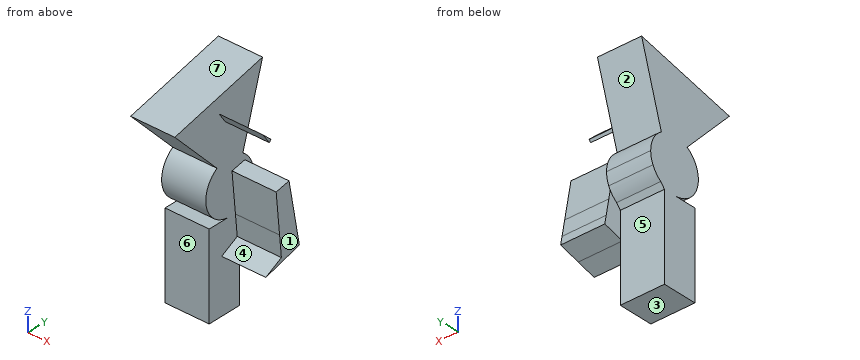
```python
from build123d import *

# Parameters (mm, degrees)
F1_DEPTH = 25.4
F3_DEPTH = 25.4


with BuildPart() as f1:
    # F0 (on Right) → F1 (new body)
    with BuildSketch(Plane.YZ):
        Polygon((-13.2883740589, -47.1408768902), (-13.2883740589, -64.2038285732), (6.5742493607, -64.2038285732), (6.5742493607, -19.7971570041), (0, -15.5264167115), (-13.2883740589, -15.5264167115), align=None)
        Polygon((0, -15.5264167115), (6.5742493607, -19.7971570041), (6.5742493607, -15.5264167115), align=None)
        with BuildLine():
            Line((0, -15.5264167115), (6.5742493607, -15.5264167115))
            Line((6.5742493607, -15.5264167115), (8.9490753187, -12.6879339074))
            ThreePointArc((8.9490753187, -12.6879339074), (4.6942234099, -14.7997933255), (0, -15.5264167115))
        make_face()
        with BuildLine():
            ThreePointArc((-8.216208845, 13.1743511459), (-14.9268228651, -4.2731224008), (0, -15.5264167115))
            ThreePointArc((0, -15.5264167115), (4.6942234099, -14.7997933255), (8.9490753187, -12.6879339074))
            Line((8.9490753187, -12.6879339074), (14.0681090783, -6.5694689939))
            ThreePointArc((14.0681090783, -6.5694689939), (15.1574559177, -3.3646910711), (15.5264167115, 0))
            ThreePointArc((15.5264167115, 0), (13.6875468883, 7.3294390017), (8.6065101962, 12.9227550523))
            Line((8.6065101962, 12.9227550523), (4.6159664635, -0.419639051))
            Line((4.6159664635, -0.419639051), (-8.216208845, 13.1743511459))
        make_face()
        with BuildLine():
            Line((14.0681090783, -6.5694689939), (8.9490753187, -12.6879339074))
            ThreePointArc((8.9490753187, -12.6879339074), (11.908257539, -9.9630827701), (14.0681090783, -6.5694689939))
        make_face()
        with BuildLine():
            Line((-35.7222311496, 42.3133387746), (-8.216208845, 13.1743511459))
            ThreePointArc((-8.216208845, 13.1743511459), (0.2321829769, 15.5246805753), (8.6065101962, 12.9227550523))
            Line((8.6065101962, 12.9227550523), (21.4547120332, 55.8807537376))
            Line((21.4547120332, 55.8807537376), (-35.7222311496, 42.3133387746))
        make_face()
        with BuildLine():
            ThreePointArc((8.6065101962, 12.9227550523), (0.2321829769, 15.5246805753), (-8.216208845, 13.1743511459))
            Line((-8.216208845, 13.1743511459), (4.6159664635, -0.419639051))
            Line((4.6159664635, -0.419639051), (8.6065101962, 12.9227550523))
        make_face()
    extrude(amount=F1_DEPTH)

    # F2 (on face) → F3 (join)
    with BuildSketch(Plane.YZ.offset(25.4)):
        Polygon((-2.8975114851, 34.5519260837), (-1.9047569793, 35.8120341569), (-6.9570055408, 40.475821833), align=None)
        Polygon((9.9313091487, 8.8122906163), (1.5386517625, 7.1337586269), (3.7782862439, -16.0091173098), (14.0347183236, -13.2288791008), align=None)
        Polygon((14.0347183236, -13.2288791008), (3.7782862439, -16.0091173098), (4.9502783877, -28.1196956248), (15.7521614301, -22.4540022549), align=None)
        Polygon((15.7521614301, -22.4540022549), (4.9502783877, -28.1196956248), (5.1841876849, -30.5367569319), (16.6601009867, -27.330934827), align=None)
        Polygon((5.1841876849, -30.5367569319), (4.9502783877, -28.1196956248), (-5.1754731685, -33.4307514131), align=None)
    extrude(amount=F3_DEPTH)


solid = f1.part
```
Verification items for the finished model (mm, model axes). Face numbers are marked on the shaded views. A direction names the side the tool comes from. Give positions to 0.01 mm unless a question says otherwise; leave off trailing zeros. Loops run counter-clockwise (first coordinate to the right, second up) from the corner with the lowest first, then second, coordinate; pieces in that order, holes last.
1. Set-up check for the marked faces 5, 6 and 7: record each of +Z, -Z, +X, -X, +Y, -Y from which the full face is reachable in a straight line by a thin tool's end or side.
2. Section check A-A, the plane x = 39.5. Enter the section's corners in (y, z), then the cut area to 3 significant figures.
3. Thickness scan on line 1 (Y direction, x = 18.5, z = -21); line 2 (X direction, y = -11, z = -5.5); line 3 (Z direction, x = 17, y = -24). Record the ranges inside material, lowest first.
4. Section check D-D, the plane y = -21. Enter the section's corners in (x, z), then the cut area to 3 significant figures.
5. Mould release check, pull along Z, two halves, no side actions. Record for the marked faces 1, 2, 3 and 4: released by +Z, released by -Z, zero draft, split by the parting line, or undercut.
6. Go/stop test with flat-tipped pins: pin 1 Ø4 at (x, y) = (14.5, -12.5) entering from +Z; pin 2 Ø1.5 at (x, z) = (12, -22.5) entering from -Y; pin 3 Ø4 at (x, y) = (17, -26) entering from -Z. Record where each tip stops, or that it passes through.
7. Section check C-C, the plane x = 23.5. Enter the section's corners in (y, z), then the cut area to 3 significant figures.
8. Section check B-B, the plane z = 38.5. Enter the section's corners in (x, y).
Geometry says:
1. face 5: -Z, -X, +Y
1. face 6: -Z, +X, -X, -Y
1. face 7: +Z, +X, -X, -Y
2. outline: (-6.96, 40.48) - (-2.9, 34.55) - (-1.9, 35.81) - close; (-5.18, -33.43) - (16.66, -27.33) - (9.93, 8.81) - (1.54, 7.13) - (4.95, -28.12) - close
2. area: 398 mm2
3. line 1: y = -13.29 to 6.57
3. line 2: x = 0 to 25.4
3. line 3: z = 29.9 to 45.09
4. outline: (0, 26.72) - (25.4, 26.72) - (25.4, 45.81) - (0, 45.81) - close
4. area: 485 mm2
5. face 1: zero draft
5. face 2: undercut
5. face 3: released by -Z
5. face 4: undercut
6. pin 1: stops at z = 48.3
6. pin 2: stops at y = -13.29
6. pin 3: stops at z = 29.9
7. outline: (-35.72, 42.31) - (-8.22, 13.17) arc R15.53 ccw to (0, -15.53) - (-13.29, -15.53) - (-13.29, -64.2) - (6.57, -64.2) - (6.57, -15.53) - (8.95, -12.69) arc R15.53 ccw to (8.61, 12.92) - (21.45, 55.88) - close
7. area: 3,080 mm2
8. outline: (0, -32.12) - (25.4, -32.12) - (25.4, -5.6) - (50.8, -5.6) - (50.8, -4.82) - (25.4, -4.82) - (25.4, 16.26) - (0, 16.26) - close
